Print and shaded views of the part. All mm, measured from the part's lowest x, y and z. Give positions to 0.01 mm unless a question says otherwise; leave off trailing zeros. Loops run counter-clockwise (first coordinate to the right, second up) from the corner with the lowest first, then second, coordinate; pieces in that order, holes last. Notation, with made-up numbers: M 19.25,14 L 24.25,14 A8 cw 24.25,26 Z; hole C 71,-8 d3. An arc over 180 degrees is marked long. Answer in a Markdown table with one row per item.
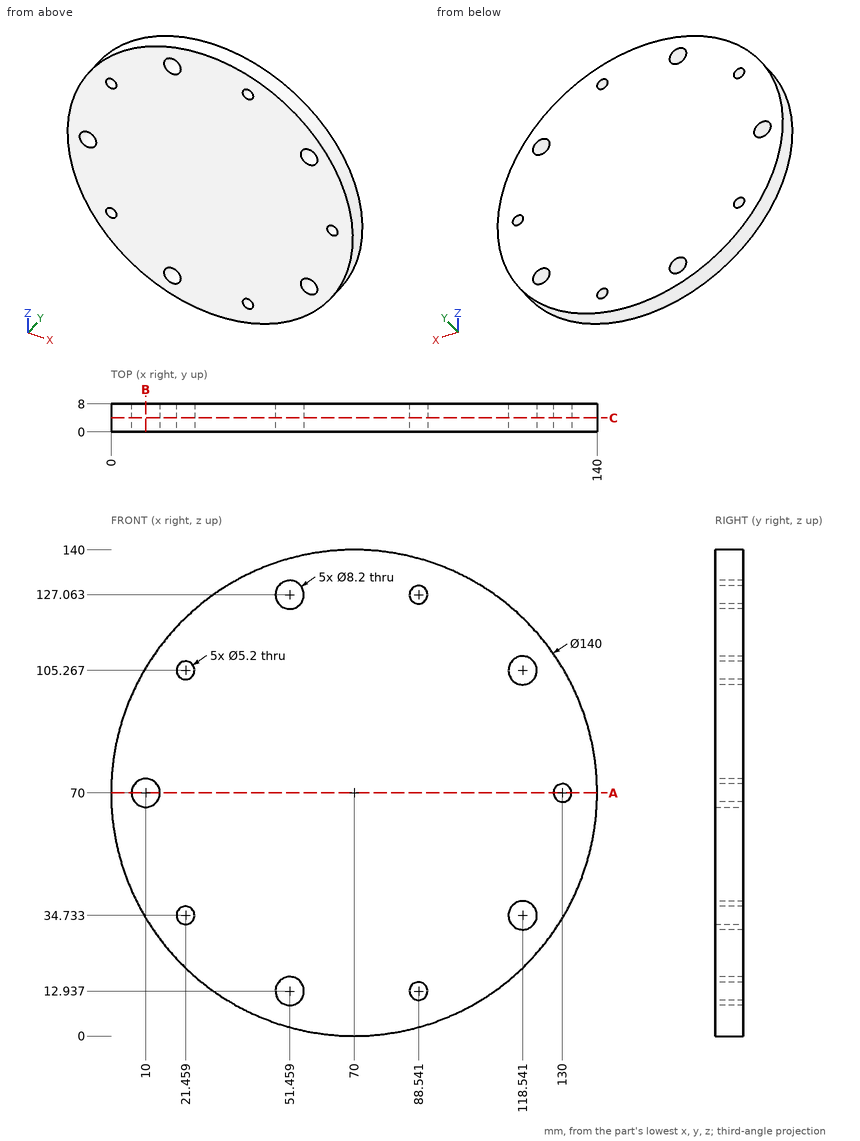
(1) Flat gauge pins, fed straight in: P1, Ø1.5, axis at x = 73, z = 34.5, coming from the -Y side; P2, Ø3, axis at y = 3.5, z = 76, coming from the -X side (1 decimal). Where does each tip first touch, or does it go through?
Established:
| item | result |
|---|---|
| P1 | stops at y = 0 |
| P2 | stops at x = 0.1 |
(2) Wall check: L1, parallel to Z at x = 55, y = 6.75 (1 decimal); L2, parallel to X at y = 6.25, z = 12.5 (1 decimal); L3, parallel to Z at x = 104, y = 1. Give the ranges that are in metal, low to high.
Established:
| item | result |
|---|---|
| L1 | z = 1.6 to 10.9, 15 to 125, 129.1 to 138.4 |
| L2 | x = 30.1 to 47.4, 55.5 to 86, 91.1 to 109.9 |
| L3 | z = 8.81 to 131.19 |
(3) Saw through at C-C, the plane y = 4. Count the separate pieces of the cut face and the enclosed holes in it, and give its area (3 significant figures).
Established:
| item | result |
|---|---|
| separate pieces | 1 |
| enclosed holes | 10 |
| area | 15,000 mm2 |
(4) Saw through at A-A, the plane z = 70. Give the cut face in (x, y).
Established:
| item | result |
|---|---|
| outline | M 0,0 L 5.9,0 L 5.9,8 L 0,8 Z; M 14.1,0 L 127.4,0 L 127.4,8 L 14.1,8 Z; M 132.6,0 L 140,0 L 140,8 L 132.6,8 Z |
(5) Saw through at B-B, the plane x = 10. Give the cut face in (y, z) (1 decimal), and give its area (3 significant figures).
Established:
| item | result |
|---|---|
| outline | M 0,33.9 L 8,33.9 L 8,65.9 L 0,65.9 Z; M 0,74.1 L 8,74.1 L 8,106.1 L 0,106.1 Z |
| area | 511 mm2 |
